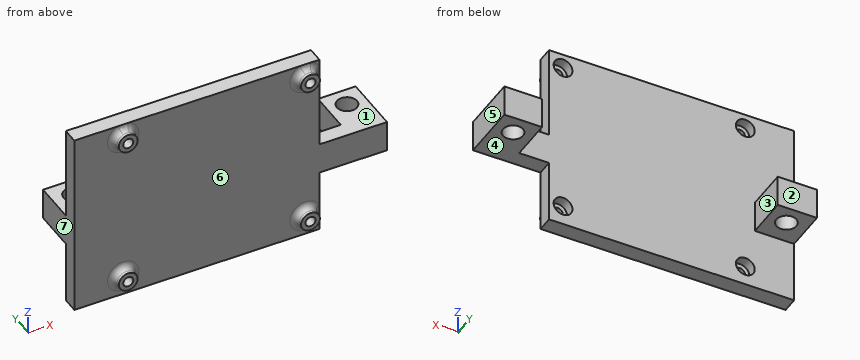
```python
from build123d import *

# Parameters (mm, degrees)
SKETCH1_R               = 3.2
BOSS_EXTRUDE1_DEPTH     = 10
SKETCH2_W               = 78
SKETCH2_H               = 5
BOSS_EXTRUDE2_DEPTH     = 30
SKETCH4_R               = 3
BOSS_EXTRUDE3_DEPTH     = 3
CUT_EXTRUDE1_REACH      = 112.623
CUT_EXTRUDE1_START      = -1.8
SKETCH4_2_R             = 3
CUT_EXTRUDE2_DEPTH      = 109.823251192
CUT_EXTRUDE2_DEPTH_BACK = 109.823251192
SKETCH3_R               = 1.6
FILLET1_R               = 2


with BuildPart() as part:
    # Sketch1 → Boss-Extrude1 (new body)
    with BuildSketch(Plane.XY):
        Polygon((99.5, 12.5), (87.5, 12.5), (87.5, -1), (12.5, -1), (12.5, 12.5), (0, 12.5), (0, -6), (99.5, -6), align=None)
        with Locations((93.5, 6.5)):
            Circle(SKETCH1_R, mode=Mode.SUBTRACT)
        with Locations((6.5, 6.5)):
            Circle(SKETCH1_R, mode=Mode.SUBTRACT)
    extrude(amount=BOSS_EXTRUDE1_DEPTH)

    # Sketch2 → Boss-Extrude2 (add, symmetric)
    with BuildSketch(Plane.XY.offset(10)):
        with Locations((39, -3.5)):
            Rectangle(SKETCH2_W, SKETCH2_H)
    extrude(amount=BOSS_EXTRUDE2_DEPTH, both=True)

    # Sketch4 → Boss-Extrude3 (add)
    with BuildSketch(Plane.XZ.offset(6)):
        with Locations(Location((15.543959644, 35.31000124, 0), (0, 0, 180))):
            Circle(SKETCH4_R)
        with Locations(Location((73.543959644, 35.31000124, 0), (0, 0, 180))):
            Circle(SKETCH4_R)
        with Locations(Location((73.543959644, -13.68999876, 0), (0, 0, 180))):
            Circle(SKETCH4_R)
        with Locations(Location((15.543959644, -13.68999876, 0), (0, 0, 180))):
            Circle(SKETCH4_R)
    extrude(amount=BOSS_EXTRUDE3_DEPTH)

    # Sketch4_2 → Cut-Extrude1 (cut, up to next)
    with BuildSketch(Plane.XZ.offset(6).offset(CUT_EXTRUDE1_START), mode=Mode.PRIVATE) as cut_extrude1_sk1:
        with Locations(Location((15.543959644, 35.31000124, 0), (0, 0, 180))):
            Circle(SKETCH4_2_R)
    cut_extrude1_tool1 = extrude(cut_extrude1_sk1.sketch, amount=-CUT_EXTRUDE1_REACH, mode=Mode.PRIVATE) & part.part
    # Sketch4_2 → Cut-Extrude1 (cut, up to next)
    with BuildSketch(Plane.XZ.offset(6).offset(CUT_EXTRUDE1_START), mode=Mode.PRIVATE) as cut_extrude1_sk2:
        with Locations(Location((73.543959644, 35.31000124, 0), (0, 0, 180))):
            Circle(SKETCH4_2_R)
    cut_extrude1_tool2 = extrude(cut_extrude1_sk2.sketch, amount=-CUT_EXTRUDE1_REACH, mode=Mode.PRIVATE) & part.part
    # Sketch4_2 → Cut-Extrude1 (cut, up to next)
    with BuildSketch(Plane.XZ.offset(6).offset(CUT_EXTRUDE1_START), mode=Mode.PRIVATE) as cut_extrude1_sk3:
        with Locations(Location((73.543959644, -13.68999876, 0), (0, 0, 180))):
            Circle(SKETCH4_2_R)
    cut_extrude1_tool3 = extrude(cut_extrude1_sk3.sketch, amount=-CUT_EXTRUDE1_REACH, mode=Mode.PRIVATE) & part.part
    # Sketch4_2 → Cut-Extrude1 (cut, up to next)
    with BuildSketch(Plane.XZ.offset(6).offset(CUT_EXTRUDE1_START), mode=Mode.PRIVATE) as cut_extrude1_sk4:
        with Locations(Location((15.543959644, -13.68999876, 0), (0, 0, 180))):
            Circle(SKETCH4_2_R)
    cut_extrude1_tool4 = extrude(cut_extrude1_sk4.sketch, amount=-CUT_EXTRUDE1_REACH, mode=Mode.PRIVATE) & part.part
    add(cut_extrude1_tool1.solids().sort_by_distance((15.54396, -4.2, 35.310001))[0], mode=Mode.SUBTRACT)
    add(cut_extrude1_tool2.solids().sort_by_distance((73.54396, -4.2, 35.310001))[0], mode=Mode.SUBTRACT)
    add(cut_extrude1_tool3.solids().sort_by_distance((73.54396, -4.2, -13.689999))[0], mode=Mode.SUBTRACT)
    add(cut_extrude1_tool4.solids().sort_by_distance((15.54396, -4.2, -13.689999))[0], mode=Mode.SUBTRACT)

    # Sketch3 → Cut-Extrude2 (cut, two sides: drawn at the far end of the back side and taken through both)
    with BuildSketch(Plane.XZ.offset(6).offset(-CUT_EXTRUDE2_DEPTH_BACK)):
        with Locations((15.543959644, 35.31000124)):
            Circle(SKETCH3_R)
        with Locations((73.543959644, 35.31000124)):
            Circle(SKETCH3_R)
        with Locations((15.543959644, -13.68999876)):
            Circle(SKETCH3_R)
        with Locations((73.543959644, -13.68999876)):
            Circle(SKETCH3_R)
    extrude(amount=CUT_EXTRUDE2_DEPTH + CUT_EXTRUDE2_DEPTH_BACK, mode=Mode.SUBTRACT)

    # Fillet1
    fillet1_edges = [part.edges().sort_by_distance(p)[0] for p in [
        (18.543959644, -6, 35.31000124),
        (76.543959644, -6, 35.31000124),
        (76.543959644, -6, -13.68999876),
        (18.543959644, -6, -13.68999876),
    ]]
    fillet(fillet1_edges, radius=FILLET1_R)


solid = part.part
```
Input: part model. Units: mm. Frame: model coordinates. Face numbers are marked on the shaded views. A direction names the side the tool comes from. Coordinates: 2 decimals unless noted, no trailing zeros. Write each loop counter-clockwise with the first axis right and the second up, starting at its lowest first coordinate (ties: lowest second). Pieces come first, ordered by that corner, then holes. Notation, with made-up numbers: (40.5, 55.25) - (94.5, 55.25) arc R8 ccw to (94.5, 61.25) - close; hole circle Ø10 at (-29.5, -14.75). An arc over 180 degrees is marked (long way). Put each result on its own line as item: value. Start each with the question number.
1) Mould query, pull axis X, two halves, no side actions, for the marked faces 4, 5, 6 and 7. Classes: pulls with the +X half, pulls with the -X half, needs draft (parallel to the pull), parting line crosses it, or undercut.
2) Contact query for flat-ended pins moving along their axis: pin 1 (5 mm diameter, centred on x = 73.54, z = 35.31, fed in from -Y); pin 2 (5 mm diameter, centred on x = 15, z = -12, fed in from +Y); pin 3 (2.5 mm diameter, centred on y = -4, z = -7, fed in from +X); pin 4 (5.5 mm diameter, centred on x = 88.5, y = 7, fed in from +Z). Output: stop coordinate, or through.
3) Cut plane D-D (x = 6.5). Return the cut outline in (y, z), plus the area to 3 significant figures.
4) Reachability of the marked faces 1, 2 and 3 from +Z, -Z, +X, -X, +Y, -Y: full face, straight path, thin tool, end or side. Return the list, or none.
5) Cut plane C-C (y = -2.75). Return the cut outline in (x, z), plus the area to 3 significant figures.
6) Cut plane A-A (x = 93.5). Return the cut outline in (y, z).
7) Ray query, L1, parallel to X at y = 3, z = 4.5; L2, parallel to Y at x = 34.5, z = 20.5; L3, parallel to X at y = -3.25, z = 31.5. Return the intervals inside material, ascending.
8) Cut plane B-B (y = 6.5). Return the cut outline in (x, z), plus the area to 3 significant figures.
Resolved:
1. face 4: needs draft
1. face 5: pulls with the +X half
1. face 6: undercut
1. face 7: pulls with the -X half
2. pin 1: stops at y = -9
2. pin 2: stops at y = -1
2. pin 3: stops at x = 78
2. pin 4: stops at z = 10
3. outline: (-6, -20) - (-1, -20) - (-1, 0) - (3.3, 0) - (3.3, 10) - (-1, 10) - (-1, 40) - (-6, 40) - close; (9.7, 0) - (12.5, 0) - (12.5, 10) - (9.7, 10) - close
3. area: 371 mm2
4. face 1: +Z, +X, +Y, -Y
4. face 2: +Z, -Z, +X, -X, +Y
4. face 3: +Z, -Z, +Y
5. outline: (0, -20) - (78, -20) - (78, 0) - (99.5, 0) - (99.5, 10) - (78, 10) - (78, 40) - (0, 40) - close; hole circle Ø6 at (15.54, -13.69); hole circle Ø6 at (15.54, 35.31); hole circle Ø6 at (73.54, -13.69); hole circle Ø6 at (73.54, 35.31)
5. area: 4,780 mm2
6. outline: (-6, 0) - (3.3, 0) - (3.3, 10) - (-6, 10) - close; (9.7, 0) - (12.5, 0) - (12.5, 10) - (9.7, 10) - close
7. L1: x = 0 to 12.5, 87.5 to 99.5
7. L2: y = -6 to -1
7. L3: x = 0 to 78
8. outline: (0, 0) - (3.3, 0) - (3.3, 10) - (0, 10) - close; (9.7, 0) - (12.5, 0) - (12.5, 10) - (9.7, 10) - close; (87.5, 0) - (90.3, 0) - (90.3, 10) - (87.5, 10) - close; (96.7, 0) - (99.5, 0) - (99.5, 10) - (96.7, 10) - close
8. area: 117 mm2
